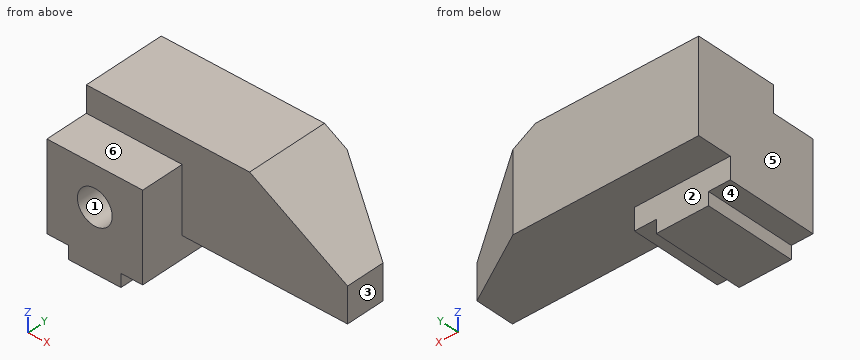
from build123d import *

# Parameters (mm, degrees)
F0_R     = 8
F3_DEPTH = 42
F4_DEPTH = 38
F5_DEPTH = 22
F7_DEPTH = 42.001


with BuildPart() as f3:
    # F0 (on Front) → F3 (new body)
    with BuildSketch(Plane.XZ):
        Polygon((10, 6), (10, 0), (34, 0), (34, 6), (44, 6), (44, 16), (44, 46), (0, 46), (0, 6), align=None)
        with Locations((22, 28)):
            Circle(F0_R, mode=Mode.SUBTRACT)
    extrude(amount=F3_DEPTH)

    # F2 (on offset) → F4 (join)
    with BuildSketch(Plane.XZ.offset(-16)):
        Polygon((75, 58), (0, 58), (0, 16), (120, 16), (120, 32.0192378865), align=None)
    extrude(amount=F4_DEPTH)

    # F5 (cut): a face of the model
    f5_faces = [f3.faces().sort_by_distance(p)[0] for p in [
        (22, -22, 28),
    ]]
    extrude(f5_faces, amount=-F5_DEPTH, mode=Mode.SUBTRACT)

    # F6 (on face) → F7 (cut, through all)
    with BuildSketch(Plane(origin=(0, 0, 16), x_dir=(1, 0, 0), z_dir=(0, 0, -1))):
        Polygon((120, 4), (85.3589838486, -16), (120, -16), align=None)
    extrude(amount=-F7_DEPTH, mode=Mode.SUBTRACT)


solid = f3.part
Geometry check sheet. Reference: the model listing, model coordinates, mm. Face numbers are marked on the shaded views. A direction names the side the tool comes from. Round coordinates to 2 decimals unless told otherwise and drop trailing zeros. Order: outer loops, then holes, each group sorted by start corner. A loop starts at its lowest first (then second) coordinate and runs counter-clockwise, first axis right, second up. Notation, with made-up numbers: M 69.5,29.5 L 127.5,29.5 A28 cw 127.5,53.5 Z; hole C 47,81.5 d8. An arc over 180 degrees is marked long. Answer in a Markdown table with one row per item.
(1) Sectioned sample at D-D, the plane y = -33. Record the cut outline in (x, z).
Responses:
| item | result |
|---|---|
| outline | M 0,6 L 10,6 L 10,0 L 34,0 L 34,6 L 44,6 L 44,46 L 0,46 Z; hole C 22,28 d16 |
(2) Sectioned sample at B-B, the plane x = 22. Record the cut outline in (y, z).
Responses:
| item | result |
|---|---|
| outline | M -42,0 L 0,0 L 0,16 L 16,16 L 16,58 L -22,58 L -22,46 L -42,46 L -42,36 L 0,36 L 0,20 L -42,20 Z |
(3) Tool access check on the marked faces 4, 5 and 6. Record the directions out of +Z, -Z, +X, -X, +Y, -Y that give a thin tool (end or side, any length) a straight path to the whole face; none if there is none.
Responses:
| item | result |
|---|---|
| face 4 | -Z, -X, +Y, -Y |
| face 5 | +Z, -Z, -X, +Y, -Y |
| face 6 | +Z, +X, -X, -Y |
(4) Go/stop test with flat-tipped pins: P1, Ø5, axis at x = 24, z = 27, coming from the -Y side; P2, Ø5, axis at x = 104.5, y = 8, coming from the -Z side (1 decimal); P3, Ø6.5, axis at y = -16, z = 4, coming from the +X side; P4, Ø2, axis at x = 56, z = 27, coming from the -Y side. Record where each tip stops, or that it passes through.
Responses:
| item | result |
|---|---|
| P1 | stops at y = 0 |
| P2 | passes through |
| P3 | stops at x = 44 |
| P4 | stops at y = -22 |
(5) Sectioned sample at C-C, the plane z = 28. Record the cut outline in (x, y).
Responses:
| item | result |
|---|---|
| outline | M 0,-42 L 14,-42 L 14,0 L 30,0 L 30,-42 L 44,-42 L 44,-22 L 120,-22 L 120,-4 L 85.36,16 L 0,16 Z |
(6) Sectioned sample at A-A, the plane y = -10.5. Record the cut outline in (x, z).
Responses:
| item | result |
|---|---|
| outline | M 0,6 L 10,6 L 10,0 L 34,0 L 34,6 L 44,6 L 44,16 L 120,16 L 120,32.02 L 75,58 L 0,58 Z; hole C 22,28 d16 |
(7) Draft check along X on the marked faces 1, 2 and 3. Enter one of: released by +X, released by -X, zero draft, split by the parting line, or undercut.
Responses:
| item | result |
|---|---|
| face 1 | undercut |
| face 2 | zero draft |
| face 3 | released by +X |
(8) Scan lines: probe 1 along X at (y, z) = (-19, 28); probe 2 along Z at (x, y) = (22, -33); probe 3 along X at (y, z) = (-26, 28). Record each from-to range of solid material in increasing order. Write a range as from..to.
Responses:
| item | result |
|---|---|
| probe 1 | x = 0..14, 30..120 |
| probe 2 | z = 0..20, 36..46 |
| probe 3 | x = 0..14, 30..44 |
